Build history of the part. All positions in model axes, mm. Face numbers are marked on the shaded views. Coordinates: 2 decimals unless noted, no trailing zeros. Write each loop counter-clockwise with the first axis right and the second up, starting at its lowest first coordinate (ties: lowest second). Pieces come first, ordered by that corner, then holes.
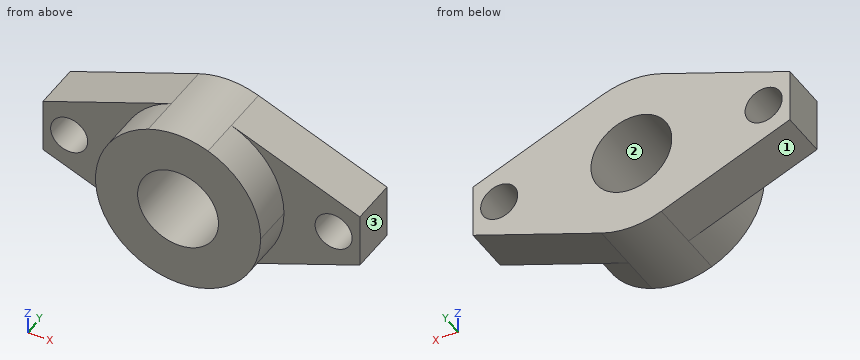
```python
from build123d import *

# Parameters (mm, degrees)
F0_R     = 6
F1_DEPTH = 13
F0_R_2   = 2.75
F2_DEPTH = 7


with BuildPart() as f1:
    # F0 (on Front) → F1 (new body)
    with BuildSketch(Plane.XZ):
        with BuildLine():
            ThreePointArc((4.442476, -11.416081), (10.11145, -6.915279), (12.25, 0))
            ThreePointArc((12.25, 0), (10.11145, 6.915279), (4.442476, 11.416081))
            ThreePointArc((4.442476, 11.416081), (0, 12.25), (-4.442476, 11.416081))
            ThreePointArc((-4.442476, 11.416081), (-12.25, 0), (-4.442476, -11.416081))
            ThreePointArc((-4.442476, -11.416081), (0, -12.25), (4.442476, -11.416081))
        make_face()
        Circle(F0_R, mode=Mode.SUBTRACT)
    extrude(amount=F1_DEPTH)

    # F0 (on Front) → F2 (join)
    with BuildSketch(Plane.XZ):
        with BuildLine():
            ThreePointArc((-4.442476, -11.416081), (-12.25, 0), (-4.442476, 11.416081))
            Line((-4.442476, 11.416081), (-23.5, 4))
            Line((-23.5, 4), (-23.5, 0))
            Line((-23.5, 0), (-23.5, -4))
            Line((-23.5, -4), (-4.442476, -11.416081))
        make_face()
        with Locations((-19.616572, 0)):
            Circle(F0_R_2, mode=Mode.SUBTRACT)
        with BuildLine():
            ThreePointArc((4.442476, 11.416081), (10.11145, 6.915279), (12.25, 0))
            ThreePointArc((12.25, 0), (10.11145, -6.915279), (4.442476, -11.416081))
            Line((4.442476, -11.416081), (23.5, -4))
            Line((23.5, -4), (23.5, 0))
            Line((23.5, 0), (23.5, 4))
            Line((23.5, 4), (4.442476, 11.416081))
        make_face()
        with Locations((19.616572, 0)):
            Circle(F0_R_2, mode=Mode.SUBTRACT)
    extrude(amount=F2_DEPTH)


solid = f1.part
```
1. Saw through at A-A on y = -4. List the corners of the cut face in (x, z), plus the area to 3 significant figures.
Computed values:
outline: (-23.5, -4) - (-4.44, -11.42) arc R12.25 ccw to (4.44, -11.42) - (23.5, -4) - (23.5, 4) - (4.44, 11.42) arc R12.25 ccw to (-4.44, 11.42) - (-23.5, 4) - close; hole circle Ø5.5 at (-19.62, 0); hole circle Ø12 at (0, 0); hole circle Ø5.5 at (19.62, 0)
area: 640 mm2
2. Mould opens along X. For the marked faces 1, 2 and 3 say: +X half, -X half, draft (parallel to the pull), parting line (faces both ways), or undercut.
Computed values:
face 1: -X half
face 2: undercut
face 3: +X half
3. Flat gauge pins, fed straight in: pin 1 (5 mm diameter, centred on x = -19.62, z = 0, fed in from +Y); pin 2 (1.5 mm diameter, centred on x = 8.5, y = -5, fed in from -Z); pin 3 (9.5 mm diameter, centred on x = 17, z = -2.5, fed in from -Y). Where does each tip first touch, or does it go through?
Computed values:
pin 1: passes through
pin 2: stops at z = -10.13
pin 3: stops at y = -7
4. Probe line 1 along X through (y, z) = (-6.5, -1.5); line 2 along Z through (x, y) = (0, -4.25); line 3 along X through (y, z) = (-6.25, 0.5). List the from-to ranges inside material, lowest first.
Computed values:
line 1: x = -23.5 to -21.92, -17.31 to -5.81, 5.81 to 17.31, 21.92 to 23.5
line 2: z = -12.25 to -6, 6 to 12.25
line 3: x = -23.5 to -22.32, -16.91 to -5.98, 5.98 to 16.91, 22.32 to 23.5
5. Saw through at C-C on y = -10.5. List the corners of the cut face in (x, z).
Computed values:
outline: (-4.44, 11.42) arc R12.25 ccw to (4.44, -11.42) arc R12.25 ccw to (12.25, 0) arc R12.25 ccw to (4.44, 11.42) arc R12.25 ccw to start; hole circle Ø12 at (0, 0)
6. Saw through at D-D on z = 5. List the corners of the cut face in (x, y), plus the area to 3 significant figures.
Computed values:
outline: (-20.93, -7) - (-11.18, -7) - (-11.18, -13) - (-3.32, -13) - (-3.32, 0) - (-20.93, 0) - close; (3.32, -13) - (11.18, -13) - (11.18, -7) - (20.93, -7) - (20.93, 0) - (3.32, 0) - close
area: 341 mm2
7. Saw through at B-B on x = 0. List the corners of the cut face in (y, z).
Computed values:
outline: (-13, -12.25) - (0, -12.25) - (0, -6) - (-13, -6) - close; (-13, 6) - (0, 6) - (0, 12.25) - (-13, 12.25) - close
